Input: part model. Units: mm. Frame: model coordinates. A direction names the side the tool comes from. Coordinates: 2 decimals unless noted, no trailing zeros. Order: outer loops, then holes, each group sorted by start corner. A loop starts at its lowest first (then second) coordinate and runs counter-clockwise, first axis right, second up. Notation, with made-up numbers: M 40,-23 L 69,-23 A16 cw 69,8 Z; hole C 29,74.5 d9. An arc over 180 degrees is marked long. One line per item, written item: value.
```python
from build123d import *

# Parameters (mm, degrees)
CHAMFER1_SIZE      = 0.48
CHAMFER1_SIZE2     = 0.831384388
CUT_EXTRUDE1_DEPTH = 2.28
DRAFT1_ANGLE       = -35
DRAFT2_ANGLE       = -8
FILLET1_R          = 0.416666667


with BuildPart() as part:
    # Sketch1 → Revolve1 (revolve)
    with BuildSketch(Plane.XY, mode=Mode.PRIVATE) as revolve1_sk:
        with BuildLine():
            Line((0, 5.75), (0, 2.4))
            Line((0, 2.4), (9.5, 2.4))
            Line((9.5, 2.4), (9.5, 0))
            Line((9.5, 0), (-3.55, 0))
            ThreePointArc((-3.55, 0), (-2.974948133, 2.694438717), (-1.35, 4.91934955))
            Line((-1.35, 4.91934955), (-1.35, 5.75))
            Line((-1.35, 5.75), (0, 5.75))
        make_face()
    revolve(revolve1_sk.sketch.rotate(Axis((-6.478309986, 0, 0), (1, 0, 0)), 90), axis=Axis((-6.478309986, 0, 0), (1, 0, 0)))

    # Chamfer1
    chamfer1_edges = [part.edges().sort_by_distance(p)[0] for p in [
        (9.5, 0, -2.4),
    ]]
    chamfer1_side = [part.faces().sort_by_distance(p)[0] for p in [
        (9.5, 0, 0),
    ]]
    chamfer(chamfer1_edges, length=CHAMFER1_SIZE, length2=CHAMFER1_SIZE2, reference=chamfer1_side[0])

    # Sketch8 → EndCone (revolve, cut)
    with BuildSketch(Plane.XY, mode=Mode.PRIVATE) as endcone_sk:
        Polygon((9.5, 0), (9.7, 0), (9.7, -2.6), (5.2, -2.6), (5.2, -2.4), align=None)
    revolve(endcone_sk.sketch.rotate(Axis((0, 0, 0), (1, 0, 0)), 270), axis=Axis((0, 0, 0), (1, 0, 0)), mode=Mode.SUBTRACT)

    # Sketch4 → Cut-Extrude1 (cut)
    with BuildSketch(Plane(origin=(-3.55, 0, 0), x_dir=(0, 0, -1), z_dir=(1, 0, 0))):
        Polygon((0.5, 2.5), (-0.5, 2.5), (-0.5, 0.5), (-2.5, 0.5), (-2.5, -0.5), (-0.5, -0.5), (-0.5, -2.5), (0.5, -2.5), (0.5, -0.5), (2.5, -0.5), (2.5, 0.5), (0.5, 0.5), align=None)
    extrude(amount=CUT_EXTRUDE1_DEPTH, mode=Mode.SUBTRACT)

    # Draft1
    draft1_faces = [part.faces().sort_by_distance(p)[0] for p in [
        (-2.160691933, 0, -2.5),
        (-2.160691933, -2.5, 0),
        (-2.160691933, 0, 2.5),
        (-2.160691933, 2.5, 0),
    ]]
    draft(draft1_faces, Plane.YZ.offset(-3.55), DRAFT1_ANGLE)

    # Draft2
    draft2_faces = [part.faces().sort_by_distance(p)[0] for p in [
        (-2.544118115, 1.102349446, -0.5),
        (-2.544118115, 0.5, -1.102349446),
        (-2.544118115, -0.5, -1.102349446),
        (-2.544118115, -1.102349446, -0.5),
        (-2.544118115, -1.102349446, 0.5),
        (-2.544118115, -0.5, 1.102349446),
        (-2.544118115, 0.5, 1.102349446),
        (-2.544118115, 1.102349446, 0.5),
    ]]
    draft(draft2_faces, Plane.YZ.offset(-3.55), DRAFT2_ANGLE)

    # Fillet1
    fillet1_edges = [part.edges().sort_by_distance(p)[0] for p in [
        (-2.391402154, 0.337169692, -0.337169692),
        (-2.391402154, 0.337169692, 0.337169692),
        (-2.391402154, -0.337169692, 0.337169692),
        (-2.391402154, -0.337169692, -0.337169692),
    ]]
    fillet(fillet1_edges, radius=FILLET1_R)


solid = part.part
```
(1) Ray query, line 1 (X direction, y = 0.25, z = 5); line 2 (Z direction, x = 8.25, y = -0.5); line 3 (X direction, y = 1, z = -3.75). Return the intervals inside material, ascending. Write a range as from..to.
Data:
line 1: x = -1.35..0
line 2: z = -0.49..0.49
line 3: x = -2.29..0
(2) Draft query along Z for faces 3 (the flat face through (-1.35, -2, -5)), 4 (the flat face through (-2.44, 1.723, -0.006)), 5 (the cylindrical face through (-0.67, -5.7, -0.75)). Return one class per face: released by +Z, released by -Z, zero draft, split by the parting line, or undercut.
Data:
face 3: zero draft
face 4: undercut
face 5: split by the parting line
(3) First-contact query: pin 1 (2 mm diameter, centred on y = 0.5, z = 0, fed in from -X); pin 2 (1.5 mm diameter, centred on y = -2.5, z = 2, fed in from -X); pin 3 (4 mm diameter, centred on y = 2.5, z = 3, fed in from +X); pin 4 (5 mm diameter, centred on x = 0, y = -3, fed in from -Z). Flat tips, straight axial feed; report the tip coordinate or a pass-through.
Data:
pin 1: stops at x = -3.49
pin 2: stops at x = -3.08
pin 3: stops at x = 6.09
pin 4: stops at z = -5.73
(4) Cut plane C-C on x = 1.25. Output: boundary loops of the cut face in (y, z), plus the area to 3 significant figures.
Data:
outline: C 0,0 d4.8
area: 18.1 mm2
(5) Access query for faces 1 (the cylindrical face through (2.636, -2.024, 1.29)), 2 (the flat face through (-2.63, 1.21, -0.37)). Directions: +Z, -Z, +X, -X, +Y, -Y. A direction counts if a zero-diameter tool reaches every point of the face in a straight line with its end or side. Return the directions, or none.
Data:
face 1: +X
face 2: -X
(6) Cut plane A-A on z = -3. Output: boundary loops of the cut face in (x, y), plus the area to 3 significant figures.
Data:
outline: M -1.35,-4.91 L 0,-4.91 L 0,4.91 L -1.35,4.91 L -1.35,3.9 A5.88 ccw -1.35,-3.9 Z
area: 21.1 mm2
(7) Cut plane B-B on y = -3.5. Output: boundary loops of the cut face in (x, z).
Data:
outline: M -1.35,-4.56 L 0,-4.56 L 0,4.56 L -1.35,4.56 L -1.35,3.46 A5.6 ccw -1.35,-3.46 Z
